Source: three-view drawing plus pictorial views. Frame: mm from the lowest corner of the part. Coordinates: 2 decimals unless noted, no trailing zeros. Write each loop counter-clockwise with the first axis right and the second up, starting at its lowest first coordinate (ties: lowest second). Pieces come first, ordered by that corner, then holes.
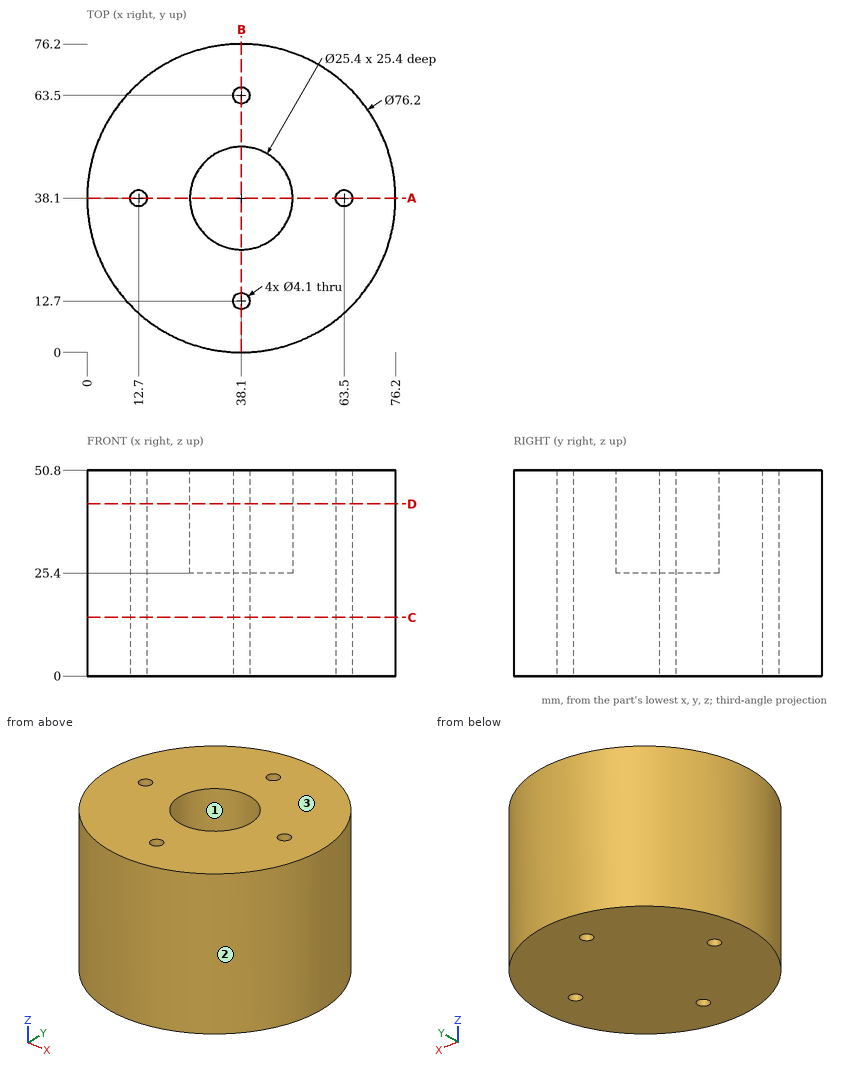
Item 1: Material intervals for line 1 (Y direction, x = 38.1, z = 29.5); line 2 (Y direction, x = 12.7, z = 13.5); line 3 (Y direction, x = 11.5, z = 32.5), sorted ascending.
Item 2: Section query D-D, the plane z = 42.5. Return loops of the section in (x, y), then the cut area to 3 significant figures.
Item 3: Pull-direction query (X, two-part tool) for the marked faces 1, 2 and 3; classes: released by +X, released by -X, zero draft, split by the parting line, or undercut.
Item 4: Section query C-C, the plane z = 14.5. Return loops of the section in (x, y).
Item 5: Pin query (flat end, axial travel): pin 1 Ø8 at (y, z) = (24.5, 15) entering from +X; pin 2 Ø6 at (y, z) = (31.5, 14) entering from +X; pin 3 Ø6 at (x, z) = (60.5, 39.5) entering from -Y; pin 4 Ø3.5 at (x, y) = (63.5, 38.1) entering from +Z. Return the tip coordinate at first contact, or that it passes through.
Item 6: Section query A-A, the plane y = 38.1. Return loops of the section in (x, z).
The answers:
1. line 1: y = 0 to 10.65, 14.75 to 25.4, 50.8 to 61.45, 65.55 to 76.2
1. line 2: y = 9.7 to 36.05, 40.15 to 66.5
1. line 3: y = 10.82 to 36.44, 39.76 to 65.38
2. outline: circle Ø76.2 at (38.1, 38.1); hole circle Ø4.1 at (12.7, 38.1); hole circle Ø25.4 at (38.1, 38.1); hole circle Ø4.1 at (38.1, 12.7); hole circle Ø4.1 at (38.1, 63.5); hole circle Ø4.1 at (63.5, 38.1)
2. area: 4,000 mm2
3. face 1: undercut
3. face 2: split by the parting line
3. face 3: zero draft
4. outline: circle Ø76.2 at (38.1, 38.1); hole circle Ø4.1 at (12.7, 38.1); hole circle Ø4.1 at (38.1, 12.7); hole circle Ø4.1 at (38.1, 63.5); hole circle Ø4.1 at (63.5, 38.1)
5. pin 1: stops at x = 74.97
5. pin 2: stops at x = 76.03
5. pin 3: stops at y = 5.31
5. pin 4: passes through
6. outline: (0, 0) - (10.65, 0) - (10.65, 50.8) - (0, 50.8) - close; (14.75, 0) - (61.45, 0) - (61.45, 50.8) - (50.8, 50.8) - (50.8, 25.4) - (25.4, 25.4) - (25.4, 50.8) - (14.75, 50.8) - close; (65.55, 0) - (76.2, 0) - (76.2, 50.8) - (65.55, 50.8) - close
